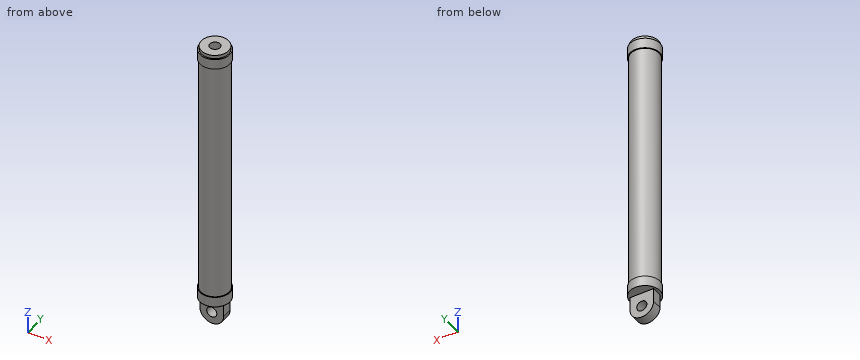
```python
from build123d import *

# Parameters (mm, degrees)
SKETCH_1_R          = 41.5
EXTRUDE_1_DEPTH     = 720
SKETCH_2_R          = 44
EXTRUDE_2_DEPTH     = 30
EXTRUDE_START       = 30
SKETCH_3_R          = 44
EXTRUDE_3_DEPTH     = 30
SKETCH_4_R          = 40
EXTRUDE_4_DEPTH     = 10
SKETCH_6_R          = 15
EXTRUDE_6_DEPTH     = 15
SKETCH_5_R          = 15
CUT_EXTRUDE_1_DEPTH = 220


with BuildPart() as part:
    # 草图1 → 拉伸1 (new body)
    with BuildSketch(Plane.XY):
        with Locations(Location((0, 0, 0), (0, 0, 180))):
            Circle(SKETCH_1_R)
    extrude(amount=EXTRUDE_1_DEPTH)

    # 草图2 → 拉伸2 (add)
    with BuildSketch(Plane.XY.offset(720)):
        Circle(SKETCH_2_R)
    extrude(amount=EXTRUDE_2_DEPTH)

    # 草图3 → 拉伸3 (add)
    with BuildSketch(Plane(origin=(0, 0, 0), x_dir=(-1, 0, 0), z_dir=(0, 0, -1)).offset(EXTRUDE_START)):
        with Locations(Location((0, 0, 0), (0, 0, 180))):
            Circle(SKETCH_3_R)
    extrude(amount=-EXTRUDE_3_DEPTH)

    # 草图4 → 拉伸4 (add)
    with BuildSketch(Plane.XY.offset(750)):
        Circle(SKETCH_4_R)
    extrude(amount=EXTRUDE_4_DEPTH)

    # 草图6 → 拉伸6 (add, symmetric)
    with BuildSketch(Plane(origin=(0, 0, 0), x_dir=(1, 0, 0), z_dir=(0, 1, 0))):
        with BuildLine():
            Line((-35, 70), (-35, 30))
            Line((-35, 30), (35, 30))
            Line((35, 30), (35, 70))
            ThreePointArc((35, 70), (0, 105), (-35, 70))
        make_face()
        with Locations(Location((0, 70, 0), (0, 0, 270))):
            Circle(SKETCH_6_R, mode=Mode.SUBTRACT)
    extrude(amount=EXTRUDE_6_DEPTH, both=True)

    # 草图5 → 切除-拉伸1 (cut)
    with BuildSketch(Plane.XY.offset(760)):
        Circle(SKETCH_5_R)
    extrude(amount=-CUT_EXTRUDE_1_DEPTH, mode=Mode.SUBTRACT)


solid = part.part
```
The model under review builds one solid part; all positions refer to its coordinate system, in mm. Give positions to 0.01 mm unless a question says otherwise; leave off trailing zeros. Write each loop counter-clockwise with the first axis right and the second up, starting at its lowest first coordinate (ties: lowest second). Pieces come first, ordered by that corner, then holes. Notation, with made-up numbers: (-18, 24.25) -> (8, 24.25) arc R19 ccw to (8, 38.25) -> close; hole circle Ø6 at (19.25, -6). An arc over 180 degrees is marked (long way). Put each result on its own line as item: value.
(1) We need section C-C, the plane z = 650.5. Give the boundary of the cut face in (x, y).
Results are:
outline: circle Ø83 at (0, 0); hole circle Ø30 at (0, 0)
(2) We need section B-B, the plane y = 0. Give the boundary of the cut face in (x, z), and give its area (3 significant figures).
Results are:
outline: (-44, -30) -> (-35, -30) -> (-35, -70) arc R35 ccw to (35, -70) -> (35, -30) -> (44, -30) -> (44, 0) -> (41.5, 0) -> (41.5, 720) -> (44, 720) -> (44, 750) -> (40, 750) -> (40, 760) -> (15, 760) -> (15, 540) -> (-15, 540) -> (-15, 760) -> (-40, 760) -> (-40, 750) -> (-44, 750) -> (-44, 720) -> (-41.5, 720) -> (-41.5, 0) -> (-44, 0) -> close; hole circle Ø30 at (0, -70)
area: 63,300 mm²
(3) We need section A-A, the plane x = 0. Give the boundary of the cut face in (y, z).
Results are:
outline: (-44, -30) -> (-15, -30) -> (-15, -55) -> (15, -55) -> (15, -30) -> (44, -30) -> (44, 0) -> (41.5, 0) -> (41.5, 720) -> (44, 720) -> (44, 750) -> (40, 750) -> (40, 760) -> (15, 760) -> (15, 540) -> (-15, 540) -> (-15, 760) -> (-40, 760) -> (-40, 750) -> (-44, 750) -> (-44, 720) -> (-41.5, 720) -> (-41.5, 0) -> (-44, 0) -> close; (-15, -105) -> (15, -105) -> (15, -85) -> (-15, -85) -> close
(4) We need section D-D, the plane z = 490.5. Give the boundary of the cut face in (x, y).
Results are:
outline: circle Ø83 at (0, 0)
(5) For pin 1 Ø3 at (y, z) = (-2, 194.5) entering from -X; pin 2 Ø24 at (x, z) = (0, -70) entering from -Y; pin 3 Ø24 at (x, y) = (0, 0) entering from -Z; pin 4 Ø24 at (y, z) = (-6, -56.5) entering from +X, all flat-tipped, find the tip position at first contact; note any pin that passes through.
Results are:
pin 1: x = -41.5
pin 2: through
pin 3: z = -105
pin 4: x = 35
(6) To check wall thickness, follow probe 1 along Y at (x, z) = (0, 585); probe 2 along Z at (x, y) = (-30.5, -31.5); probe 3 along X at (y, z) = (4.25, -70). State the ranges of each line that lie inside material, in increasing order. Write a range as from..to.
Results are:
probe 1: -41.5..-15, 15..41.5
probe 2: -30..0, 720..750
probe 3: -35..-15, 15..35
